Read the model definition and answer for the solid it produces. Units are mm, in the model's axes. A direction names the side the tool comes from. Give positions to 0.01 mm unless a question says otherwise; leave off trailing zeros. Loops run counter-clockwise (first coordinate to the right, second up) from the corner with the lowest first, then second, coordinate; pieces in that order, holes last.
(1) Determine the mould class of faces 3 (the face through (-73.613, -34.112, 1.565)), 4 (the face through (-4.19, 21.76, 1.57)), 5 (the face through (9.485, -66.301, 4.785)) for opening direction Y: pulls with the +Y half, pulls with the -Y half, needs draft (parallel to the pull), parting line crosses it, or undercut.
(2) Find section B-B, the plane z = 1. Write down the section's boundary in (x, y).
(3) Which of the six approach directions +Z, -Z, +X, -X, +Y, -Y give full straight-line access (tool end or side, diameter ignored) to faces 1 (the face through (8.56, 13.44, 1.57)), 2 (the face through (-72.785, -18.916, 4.785))?
(4) Each of these flat-tipped pins is pushed along its axis until it touches: P1, Ø2, axis at y = -71.5, z = 3.5, coming from the +X side; P2, Ø5, axis at x = -2.5, y = 21.5, coming from the +Z side. Where does it stop, or does it pass through?
(5) Straight lines are drawn through the part: probe 1 along X at (y, z) = (9.5, 2.75); probe 2 along Y at (x, z) = (-85, 2.5); probe 3 along Y at (x, z) = (-24.5, 1). For each, find the intervals that lie inside material, in ascending order.
```python
from build123d import *

# Parameters (mm, degrees)
F1_DEPTH = 6.35
F2_SIZE  = 3.17499


# Not quite as in the source:
# - a fillet or chamfer is up to 0.001 mm smaller than in the source, because OpenCascade refuses the exact size


with BuildPart() as f1:
    # F0 (on Top) → F1 (new body)
    with BuildSketch(Plane.XY):
        with BuildLine():
            Line((-17.3524573698, -16.6459077914), (19.1028173324, 47.7399711053))
            Line((19.1028173324, 47.7399711053), (-29.8718068032, -2.0647344031))
            ThreePointArc((-29.8718068032, -2.0647344031), (-28.46767213, -4.137767395), (-27.974045361, -6.5924349039))
            ThreePointArc((-27.974045361, -6.5924349039), (-28.8114925566, -9.7443012682), (-31.1029466457, -12.0648222317))
            Line((-31.1029466457, -12.0648222317), (-28.352068997, -16.7383418336))
            ThreePointArc((-28.352068997, -16.7383418336), (-22.8646469969, -15.2184562862), (-17.3524573698, -16.6459077914))
        make_face()
        with BuildLine():
            ThreePointArc((-31.1029466457, -12.0648222317), (-36.70470147, -12.4792826589), (-40.4436473061, -8.2874192794))
            Line((-40.4436473061, -8.2874192794), (-107.7592687025, -26.9322474098))
            Line((-107.7592687025, -26.9322474098), (-33.7718245819, -26.3105019555))
            ThreePointArc((-33.7718245819, -26.3105019555), (-32.3443730767, -20.7983123285), (-28.352068997, -16.7383418336))
            Line((-28.352068997, -16.7383418336), (-31.1029466457, -12.0648222317))
        make_face()
        with BuildLine():
            Line((-33.7718245819, -26.3105019555), (-107.7592687025, -26.9322474098))
            Line((-107.7592687025, -26.9322474098), (-40.1398164365, -44.4431632978))
            ThreePointArc((-40.1398164365, -44.4431632978), (-36.4718453922, -40.1890566965), (-30.8639164155, -40.5093177627))
            Line((-30.8639164155, -40.5093177627), (-28.1919685396, -35.7902280353))
            ThreePointArc((-28.1919685396, -35.7902280353), (-32.2519390345, -31.7979239556), (-33.7718245819, -26.3105019555))
        make_face()
        with BuildLine():
            Line((20.339812506, -99.4619274356), (-17.1923569125, -35.6977939932))
            ThreePointArc((-17.1923569125, -35.6977939932), (-22.6797789126, -37.2176795405), (-28.1919685396, -35.7902280353))
            Line((-28.1919685396, -35.7902280353), (-30.8639164155, -40.5093177627))
            ThreePointArc((-30.8639164155, -40.5093177627), (-28.5067207601, -42.8369871561), (-27.6425935032, -46.0350647422))
            ThreePointArc((-27.6425935032, -46.0350647422), (-28.1158002373, -48.440433926), (-29.4648930024, -50.4873033))
            Line((-29.4648930024, -50.4873033), (20.339812506, -99.4619274356))
        make_face()
        with BuildLine():
            ThreePointArc((1.6949843755, -32.1463060392), (-3.8231655338, -31.0968032352), (-6.3497758029, -26.0800637457))
            Line((-6.3497758029, -26.0800637457), (-11.7726013276, -26.1256338712))
            ThreePointArc((-11.7726013276, -26.1256338712), (-11.7723100484, -26.1718504844), (-11.7722129547, -26.2180679134))
            ThreePointArc((-11.7722129547, -26.2180679134), (-13.2229088841, -31.6779938989), (-17.1923569125, -35.6977939932))
            Line((-17.1923569125, -35.6977939932), (20.339812506, -99.4619274356))
            Line((20.339812506, -99.4619274356), (1.6949843755, -32.1463060392))
        make_face()
        with BuildLine():
            Line((1.5919014444, -19.8794811608), (19.1028173324, 47.7399711053))
            Line((19.1028173324, 47.7399711053), (-17.3524573698, -16.6459077914))
            ThreePointArc((-17.3524573698, -16.6459077914), (-13.2924868749, -20.6382118711), (-11.7726013276, -26.1256338712))
            Line((-11.7726013276, -26.1256338712), (-6.3497758029, -26.0800637457))
            ThreePointArc((-6.3497758029, -26.0800637457), (-3.9078316495, -21.0215715485), (1.5919014444, -19.8794811608))
        make_face()
    extrude(amount=F1_DEPTH)

    # F2 (size 3.175 in the source; OpenCascade refuses exactly that, so slightly less here)
    f2_edges = [f1.edges().sort_by_distance(p)[0] for p in [
        (-74.101458, -17.609833, 6.35),
        (-73.949543, -35.687705, 6.35),
        (-73.949543, -35.687705, 0),
        (-4.56254, -74.974615, 6.35),
        (11.017398, -65.804117, 6.35),
        (-5.384495, 22.837618, 6.35),
        (-74.101458, -17.609833, 0),
        (-4.56254, -74.974615, 0),
        (11.017398, -65.804117, 0),
        (-5.384495, 22.837618, 0),
        (10.347359, 13.930245, 0),
        (10.347359, 13.930245, 6.35),
    ]]
    chamfer(f2_edges, length=F2_SIZE)


solid = f1.part
```
Entries:
1. face 3: pulls with the -Y half
1. face 4: pulls with the +Y half
1. face 5: undercut
2. outline: (-99.36, -26.86) - (-39.22, -42.43) arc R6.35 cw to (-28.21, -48.67) - (16.08, -92.22) - (-0.5, -32.36) arc R6.35 cw to (-0.61, -19.71) - (14.96, 40.43) - (-28.59, -3.86) arc R6.35 cw to (-39.49, -10.28) - close; hole (-11.77, -26.22) arc R11 ccw to (-11.77, -26.13) arc R11 ccw (long way) to start
3. face 1: -Z, +X
3. face 2: +Z, -X, +Y
4. P1: stops at x = 12.86
4. P2: stops at z = 6.35
5. probe 1: x = -17.9 to 8.76
5. probe 2: y = -32.13 to -21.33
5. probe 3: y = -52.32 to -37.08, -15.35 to 0.3
